For this review, take the finished solid that the model builds, in its own axes (mm). Face numbers are marked on the shaded views. A direction names the side the tool comes from. Round coordinates to 2 decimals unless told otherwise and drop trailing zeros. Order: outer loops, then holes, each group sorted by start corner. A loop starts at its lowest first (then second) coordinate and runs counter-clockwise, first axis right, second up. Notation, with made-up numbers: M 86,59 L 135,59 A29 cw 135,81 Z; hole C 51,-15 d8. An arc over 180 degrees is marked long. Answer in a Markdown table with one row per item. Add a question column.
```python
from build123d import *

# Parameters (mm, degrees)
F0_W     = 40
F0_H     = 200
F1_DEPTH = 3
F2_W     = 3
F2_H     = 200
F3_DEPTH = 40
F5_DEPTH = 100


with BuildPart() as f1:
    # F0 (on Front) → F1 (new body)
    with BuildSketch(Plane.XZ):
        Rectangle(F0_W, F0_H)
    extrude(amount=F1_DEPTH)

    # F2 (on Front) → F3 (join)
    with BuildSketch(Plane.XZ):
        with Locations((21.5, 0)):
            Rectangle(F2_W, F2_H)
    extrude(amount=F3_DEPTH)

    # F4 (on Top) → F5 (join, symmetric)
    with BuildSketch(Plane.XY):
        Polygon((10, -3), (20, -13), (20, -3), align=None)
    extrude(amount=F5_DEPTH, both=True)


solid = f1.part
```
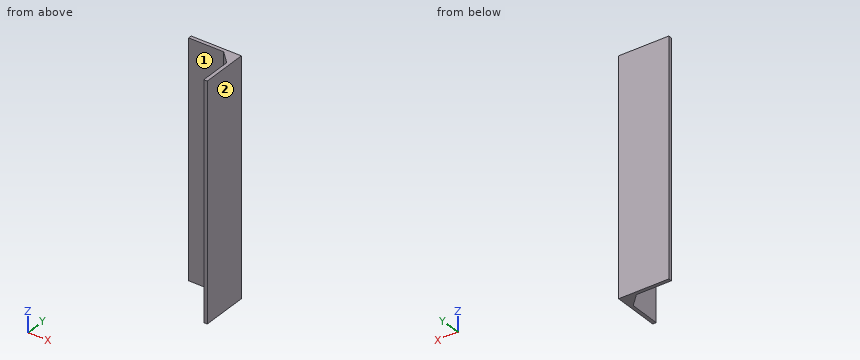
1. For the marked faces 1 and 2, list the 3-axis set-ups (+Z, -Z, +X, -X, +Y, -Y) from which the entire face can be reached by the end or side of a thin tool; tool diameter is ignored.
2. Clearance check with flat-ended pins moving along their axes: pin 1 Ø6 at (y, z) = (-32, 43) entering from -X; pin 2 Ø10 at (x, z) = (-4.5, 54) entering from -Y; pin 3 Ø3 at (x, z) = (16, 78) entering from -Y. State where each tip first meets the part, or that it passes through.
3. To check wall thickness, follow probe 1 along X at (y, z) = (-36, 56.5); probe 2 along Y at (x, z) = (-9, 30); probe 3 along X at (y, z) = (-5, -79). State the ranges of each line that lie inside material, in increasing order. Write a range as [from, to].
4. Consider section A-A on z = 13.5. Write out the cut boundary in (x, y).
5. Consider section C-C on x = -15. Write out the cut boundary in (y, z).
6. Consider section B-B on y = -7. Write out the cut boundary in (x, z), plus the area to 3 significant figures.
Solved:
| question | item | result |
|---|---|---|
| 1 | face 1 | +Z, -Z, -X, -Y |
| 1 | face 2 | +Z, -Z, +X, +Y, -Y |
| 2 | pin 1 | stops at x = 20 |
| 2 | pin 2 | stops at y = -3 |
| 2 | pin 3 | stops at y = -10.5 |
| 3 | probe 1 | x = [20, 23] |
| 3 | probe 2 | y = [-3, 0] |
| 3 | probe 3 | x = [12, 23] |
| 4 | outline | M -20,-3 L 10,-3 L 20,-13 L 20,-40 L 23,-40 L 23,0 L -20,0 Z |
| 5 | outline | M -3,-100 L 0,-100 L 0,100 L -3,100 Z |
| 6 | outline | M 14,-100 L 23,-100 L 23,100 L 14,100 Z |
| 6 | area | 1,800 mm^2 |
